from build123d import *

# Parameters (mm, degrees)
SKETCH2_W               = 60
SKETCH2_H               = 60
BOSS_EXTRUDE1_DEPTH     = 500
SHELL1_T                = -5
SKETCH3_W               = 100
SKETCH3_H               = 50
SKETCH3_W_2             = 50
CUT_EXTRUDE1_DEPTH      = 505.479930225
CUT_EXTRUDE3_DEPTH      = 504.909714135
CUT_EXTRUDE3_DEPTH_BACK = 504.909714135
SKETCH4_R               = 15


with BuildPart() as part:
    # Sketch2 → Boss-Extrude1 (new body)
    with BuildSketch(Plane(origin=(0, 0, 0), x_dir=(-1, 0, 0), z_dir=(0, 1, 0))):
        Rectangle(SKETCH2_W, SKETCH2_H)
    extrude(amount=BOSS_EXTRUDE1_DEPTH)

    # Shell1
    shell1_openings = [part.faces().sort_by_distance(p)[0] for p in [
        (0, 500, 0),
        (0, 0, 0),
    ]]
    offset(amount=SHELL1_T, openings=shell1_openings, kind=Kind.INTERSECTION)

    # Sketch3 → Cut-Extrude1 (cut, through all)
    with BuildSketch(Plane.YZ.offset(30)):
        with Locations((50, 0)):
            Rectangle(SKETCH3_W, SKETCH3_H)
        with Locations((475, 0)):
            Rectangle(SKETCH3_W_2, SKETCH3_H)
    extrude(amount=-CUT_EXTRUDE1_DEPTH, mode=Mode.SUBTRACT)

    # Sketch4 → Cut-Extrude3 (cut, two sides: drawn at the far end of the back side and taken through both)
    with BuildSketch(Plane(origin=(0, 0, 25), x_dir=(1, 0, 0), z_dir=(0, 0, -1)).offset(-CUT_EXTRUDE3_DEPTH_BACK)):
        with Locations(Location((0, -50, 0), (0, 0, 180))):
            Circle(SKETCH4_R)
    extrude(amount=CUT_EXTRUDE3_DEPTH + CUT_EXTRUDE3_DEPTH_BACK, mode=Mode.SUBTRACT)


solid = part.part
Work out the finished part from the listing and answer in its coordinate system (mm). A direction names the side the tool comes from. Give positions to 0.01 mm unless a question says otherwise; leave off trailing zeros. Loops run counter-clockwise (first coordinate to the right, second up) from the corner with the lowest first, then second, coordinate; pieces in that order, holes last. Notation, with made-up numbers: (51, 66.25) -> (91, 66.25) arc R24 cw to (91, 77.25) -> close; hole circle Ø2 at (16, 31). An arc over 180 degrees is marked (long way). Use a Markdown table: item, result. Add a question column.
1) The part is cut by section B-B, the plane x = 0. Determine the outline of the cut face in (y, z).
2) Each of these flat-tipped pins is pushed along its axis until it touches: P1, Ø1.5, axis at x = 28, z = 5, coming from the -Y side; P2, Ø18, axis at x = 0, y = 50, coming from the +Z side; P3, Ø2.5, axis at x = -27.5, z = 3, coming from the +Y side; P4, Ø8, axis at y = 96.5, z = 17.5, coming from the -X side. Where does it stop, or does it pass through?
3) For a pull along Z with two mould halves and no side action, classify faces 3 (the flat face through (30, 246, 0)), 4 (the flat face through (0, 247, 25)), 5 (the flat face through (25, 273, 0)), 6 (the flat face through (0, 246, 30)) as +Z half, -Z half, draft (parallel to the pull), parting line (faces both ways), or undercut.
4) The part is cut by section D-D, the plane y = 232. Determine the outline of the cut face in (x, z), plus the area to 3 significant figures.
5) Which of the six approach directions +Z, -Z, +X, -X, +Y, -Y give full straight-line access (tool end or side, diameter ignored) to faces 1 (the flat face through (-25, 273, 0)), 2 (the cylindrical face through (1.953, 64.872, 27.535))?
6) The part is cut by section A-A, the plane y = 50. Determine the outline of the cut face in (x, z).
7) Consider line 1 along X through (y, z) = (300.5, 9.5); line 2 along X through (y, z) = (50, 26.7). Determine where each line is inside the solid, lowest interval first.
8) The part is cut by section C-C, the plane z = 13. Determine the outline of the cut face in (x, y), plus the area to 3 significant figures.
Reported:
| question | item | result |
|---|---|---|
| 1 | outline | (0, -30) -> (35, -30) -> (35, -25) -> (0, -25) -> close; (0, 25) -> (35, 25) -> (35, 30) -> (0, 30) -> close; (65, -30) -> (500, -30) -> (500, -25) -> (65, -25) -> close; (65, 25) -> (500, 25) -> (500, 30) -> (65, 30) -> close |
| 2 | P1 | stops at y = 100 |
| 2 | P2 | passes through |
| 2 | P3 | stops at y = 450 |
| 2 | P4 | stops at x = -30 |
| 3 | face 3 | draft |
| 3 | face 4 | undercut |
| 3 | face 5 | undercut |
| 3 | face 6 | +Z half |
| 4 | outline | (-30, -30) -> (30, -30) -> (30, 30) -> (-30, 30) -> close; hole (-25, -25) -> (25, -25) -> (25, 25) -> (-25, 25) -> close |
| 4 | area | 1,100 mm^2 |
| 5 | face 1 | +Y, -Y |
| 5 | face 2 | +Z, -Z |
| 6 | outline | (-30, -30) -> (-15, -30) -> (-15, -25) -> (-30, -25) -> close; (-30, 25) -> (-15, 25) -> (-15, 30) -> (-30, 30) -> close; (15, -30) -> (30, -30) -> (30, -25) -> (15, -25) -> close; (15, 25) -> (30, 25) -> (30, 30) -> (15, 30) -> close |
| 7 | line 1 | x = -30 to -25, 25 to 30 |
| 7 | line 2 | x = -30 to -15, 15 to 30 |
| 8 | outline | (-30, 100) -> (-25, 100) -> (-25, 450) -> (-30, 450) -> close; (25, 100) -> (30, 100) -> (30, 450) -> (25, 450) -> close |
| 8 | area | 3,500 mm^2 |
